Part model, mm, in its own coordinate system. Give positions to 0.01 mm unless a question says otherwise; leave off trailing zeros. Order: outer loops, then holes, each group sorted by start corner. A loop starts at its lowest first (then second) coordinate and runs counter-clockwise, first axis right, second up. Notation, with made-up numbers: (35.5, 5.5) -> (43.5, 5.5) arc R19 cw to (43.5, 38.5) -> close; hole circle Ø11 at (27.5, 7). An arc over 180 degrees is marked (long way). Write item = value, one per line. Start each with the question number.
(1) Probe line 1 along X through (y, z) = (0.35, 31.75); line 2 along X through (y, z) = (2.1, 31.75); line 3 along Z through (x, y) = (-5.08, 0.55). List the from-to ranges inside material, lowest first. Write a range as from..to.
(2) Saw through at C-C, the plane z = 31.75. State how many separate pieces and enclosed holes the cut face has, then the cut area to 3 significant figures.
(3) Saw through at A-A, the plane x = -68.5. List the corners of the cut face in (y, z) (3 decimals).
(4) Saw through at B-B, the plane z = 48. List the corners of the cut face in (x, y) (3 decimals), then the cut area to 3 significant figures.
(5) Saw through at D-D, the plane y = 7.25. List the corners of the cut face in (x, z) (3 decimals).
(6) Flat gauge pins, fed straight in: pin 1 (7.5 mm diameter, centred on x = -27.5, y = 10, fed in from -Z); pin 2 (2 mm diameter, centred on x = -23, y = 6.5, fed in from -Z); pin 3 (6 mm diameter, centred on x = -48, z = 8, fed in from +Y) (3 decimals). Where does each tip first touch, or does it go through?
Autodesk Inventor part; units mm, degrees
ref_plane "YZ Plane" through (0, 0, 0) normal (1, 0, 0) x (0, 1, 0)
ref_plane "XZ Plane" through (0, 0, 0) normal (0, 1, 0) x (-1, 0, 0)
ref_plane "XY Plane" through (0, 0, 0) normal (0, 0, 1) x (1, 0, 0)
sketch "Sketch1" plane through (0, 0, 0) normal (0, 1, 0) x (-1, 0, 0)
  line L0 (0, 0) -> (83.82, 0)
  line L1 (83.82, 0) -> (83.82, 63.5)
  line L2 (83.82, 63.5) -> (0, 63.5)
  line L3 (0, 63.5) -> (0, 0)
  line L4 (73.66, 53.975) -> (58.42, 53.975)
  line L5 (58.42, 53.975) -> (58.42, 9.525)
  line L6 (58.42, 9.525) -> (73.66, 9.525)
  line L7 (73.66, 9.525) -> (73.66, 53.975)
  line L8 (49.53, 53.975) -> (34.29, 53.975)
  line L9 (34.29, 53.975) -> (34.29, 9.525)
  line L10 (34.29, 9.525) -> (49.53, 9.525)
  line L11 (49.53, 9.525) -> (49.53, 53.975)
  line L12 (25.4, 53.975) -> (10.16, 53.975)
  line L13 (10.16, 53.975) -> (10.16, 9.525)
  line L14 (10.16, 9.525) -> (25.4, 9.525)
  line L15 (25.4, 9.525) -> (25.4, 53.975)
  dimension "d0" = 83.82
  dimension "d1" = 63.5
  dimension "d41" = 10.16
  dimension "d42" = 8.89
  dimension "d43" = 8.89
  dimension "d44" = 15.24
  dimension "d45" = 15.24
  dimension "d46" = 15.24
extrude "Extrusion1" add sketch "Sketch1" along normal blind 3.175
sketch "Sketch4" plane through (0, 3.175, 0) normal (0, 1, 0) x (1, 0, 0)
  line L0 (-83.82, -63.5) -> (0, -63.5)
  line L1 (0, 0) -> (-83.82, 0)
  line L2 (-66.675, 0) -> (-57.15, 0)
  line L3 (-57.15, 0) -> (-57.15, -3.9624)
  line L4 (-57.15, -3.9624) -> (-66.675, -3.9624)
  line L5 (-66.675, -3.9624) -> (-66.675, 0)
  line L6 (-31.75, 0) -> (-22.225, 0)
  line L7 (-22.225, 0) -> (-22.225, -3.9624)
  line L8 (-22.225, -3.9624) -> (-31.75, -3.9624)
  line L9 (-31.75, -3.9624) -> (-31.75, 0)
  line L10 (-66.675, -63.5) -> (-57.15, -63.5)
  line L11 (-57.15, -63.5) -> (-57.15, -59.5376)
  line L12 (-57.15, -59.5376) -> (-66.675, -59.5376)
  line L13 (-66.675, -59.5376) -> (-66.675, -63.5)
  line L14 (-31.75, -63.5) -> (-22.225, -63.5)
  line L15 (-22.225, -63.5) -> (-22.225, -59.5376)
  line L16 (-22.225, -59.5376) -> (-31.75, -59.5376)
  line L17 (-31.75, -59.5376) -> (-31.75, -63.5)
extrude "Extrusion4" add sketch "Sketch4" along normal blind 11.1252
sketch "Sketch5" plane through (-22.225, 3.175, 63.5) normal (1, 0, 0) x (0, 0, -1)
  line L0 (3.9624, 0) -> (0, 0)
  line L1 (3.9624, 0) -> (3.9624, 11.1252)
  line L2 (0, 11.1252) -> (3.9624, 11.1252)
  line L3 (0, 0) -> (0, 11.1252)
  line L4 (3.9624, 12.7) -> (2.1844, 12.7)
  line L5 (3.9624, -0.6232) -> (0.7874, -0.6232)
  line L6 (2.1844, 11.1252) -> (0.7874, 0)
  line L7 (0.7874, 0) -> (0, 0)
  line L8 (0, 0) -> (0, 11.1252)
  line L9 (0, 11.1252) -> (2.1844, 11.1252)
  line L10 (59.5376, 0) -> (63.5, 0)
  line L11 (59.5376, 0) -> (59.5376, 11.1252)
  line L12 (63.5, 11.1252) -> (59.5376, 11.1252)
  line L13 (63.5, 0) -> (63.5, 11.1252)
  line L14 (59.5376, 12.7) -> (61.3156, 12.7)
  line L15 (59.5376, -0.6232) -> (62.7126, -0.6232)
  line L16 (61.3156, 11.1252) -> (62.7126, 0)
  line L17 (62.7126, 0) -> (63.5, 0)
  line L18 (63.5, 0) -> (63.5, 11.1252)
  line L19 (63.5, 11.1252) -> (61.3156, 11.1252)
  point P0 (63.5, -3.175)
  dimension "d17" = 1.778
  dimension "d18" = 3.175
extrude "Extrusion5" cut sketch "Sketch5" against normal blind 44.45 contours L0 L3 L2 L6 | L16 L12 L13 L10
fillet "Fillet1" radius 3.175 4 edges at (-61.9125, 3.175, 62.7126) (-26.9875, 3.175, 62.7126) (-26.9875, 3.175, 0.7874) (-61.9125, 3.175, 0.7874)
sketch "Sketch6" plane through (0, 14.3002, 0) normal (0, 1, 0) x (1, 0, 0)
  line L0 (-22.225, -59.5376) -> (-31.75, -59.5376)
  line L1 (-31.75, -59.5376) -> (-22.225, -59.5376)
  line L2 (-22.225, -59.5376) -> (-22.225, -57.912)
  line L3 (-22.225, -57.912) -> (-31.75, -57.912)
  line L4 (-31.75, -57.912) -> (-31.75, -59.5376)
  line L5 (-57.15, -59.5376) -> (-66.675, -59.5376)
  line L6 (-66.675, -59.5376) -> (-66.675, -57.912)
  line L7 (-66.675, -57.912) -> (-57.15, -57.912)
  line L8 (-57.15, -57.912) -> (-57.15, -59.5376)
  line L9 (-31.75, -2.1844) -> (-22.225, -2.1844)
  line L10 (-22.225, -2.1844) -> (-22.225, -3.9624)
  line L11 (-22.225, -3.9624) -> (-31.75, -3.9624)
  line L12 (-31.75, -3.9624) -> (-31.75, -2.1844)
  line L13 (-31.75, -3.9624) -> (-22.225, -3.9624)
  line L14 (-22.225, -3.9624) -> (-22.225, -5.588)
  line L15 (-22.225, -5.588) -> (-31.75, -5.588)
  line L16 (-31.75, -5.588) -> (-31.75, -3.9624)
  line L17 (-57.15, -3.9624) -> (-66.675, -3.9624)
  line L18 (-66.675, -3.9624) -> (-66.675, -5.588)
  line L19 (-66.675, -5.588) -> (-57.15, -5.588)
  line L20 (-57.15, -5.588) -> (-57.15, -3.9624)
  line L21 (-66.675, -3.9624) -> (-57.15, -3.9624)
  point P0 (0, 0)
  dimension "d50" = 1.6256
  dimension "d51" = 1.6256
  dimension "d52" = 1.6256
  dimension "d53" = 1.6256
  dimension "d54" = 0
extrude "Extrusion6" add sketch "Sketch6" against normal blind 1.6002 contours L0 L4 L3 L2 | L5 L6 L7 L8 | L11 L14 L15 L16 | L20 L19 L18 L17
sketch "Sketch7" plane through (-22.225, 3.175, 63.5) normal (1, 0, 0) x (0, 0, -1)
  line L0 (5.588, 11.1252) -> (5.588, 9.525)
  line L1 (2.1844, 11.1252) -> (5.588, 11.1252)
  line L2 (4.5974, 11.1252) -> (5.588, 9.525)
  line L3 (4.5974, 11.1252) -> (5.588, 11.1252)
  line L4 (5.588, 9.525) -> (5.588, 11.1252)
  line L5 (61.3156, 11.1252) -> (62.4649, 1.9722)
  arc A0 (62.4649, 1.9722) -> (63.5, 0) centre (65.6152, 2.3678) ccw
  line L6 (59.5376, 0) -> (63.5, 0)
  line L7 (59.5376, 0) -> (59.5376, 9.525)
  line L8 (57.15, 9.525) -> (59.5376, 9.525)
  line L9 (57.15, 11.1252) -> (57.15, 9.525)
  line L10 (61.3156, 11.1252) -> (57.15, 11.1252)
  line L11 (58.9026, 11.1252) -> (57.15, 9.525)
  line L12 (58.9026, 11.1252) -> (57.15, 11.1252)
  line L13 (57.15, 9.525) -> (57.15, 11.1252)
  point P0 (63.5, -3.175)
extrude "Extrusion7" cut sketch "Sketch7" against normal blind 44.45 contours L0 L2 L1 | L11 L9 L10
sketch "Sketch8" plane through (0, 3.175, 0) normal (0, 1, 0) x (1, 0, 0)
  circle A0 centre (-79.0956, -31.75) radius 3.175
  circle A1 centre (-5.08, -31.75) radius 3.1695
  line L0 (0, -63.5) -> (0, 0)
  line L1 (-66.675, 0) -> (-83.82, 0)
  line L2 (0, 0) -> (-22.225, 0)
  dimension "d29" = 74.0156
  dimension "d47" = 5.08
  dimension "d48" = 31.75
  dimension "d49" = 31.75
extrude "Extrusion8" cut sketch "Sketch8" against normal blind 1.905
sketch "Sketch9" plane through (0, 3.175, 0) normal (0, 1, 0) x (1, 0, 0)
  circle A0 centre (-5.08, -31.75) radius 3.1695
  circle A1 centre (-79.0956, -31.75) radius 3.175
  circle A2 centre (-79.0956, -31.75) radius 1.5875
  circle A3 centre (-5.08, -31.75) radius 1.5875
extrude "Extrusion9" cut sketch "Sketch9" against normal blind 3.175 contours A2 | A3
sketch "Sketch12" plane through (0, 12.7, 0) normal (0, -1, 0) x (1, 0, 0)
  line L0 (-22.225, 3.9624) -> (-22.225, 5.588)
  line L1 (-22.225, 5.588) -> (-31.75, 5.588)
  line L2 (-22.225, 3.9624) -> (-31.75, 3.9624)
  line L3 (-31.75, 3.9624) -> (-31.75, 5.588)
  line L4 (-31.75, 5.588) -> (-22.225, 5.588)
  line L5 (-22.225, 5.588) -> (-22.225, 3.9624)
  line L6 (-57.15, 3.9624) -> (-66.675, 3.9624)
  line L7 (-57.15, 5.588) -> (-66.675, 5.588)
  line L8 (-57.15, 3.9624) -> (-66.675, 3.9624)
  line L9 (-66.675, 3.9624) -> (-66.675, 5.588)
  line L10 (-66.675, 5.588) -> (-57.15, 5.588)
  line L11 (-57.15, 5.588) -> (-57.15, 3.9624)
  line L12 (-66.675, 57.912) -> (-57.15, 57.912)
  line L13 (-57.15, 59.5376) -> (-66.675, 59.5376)
  line L14 (-66.675, 59.5376) -> (-66.675, 57.912)
  line L15 (-66.675, 57.912) -> (-57.15, 57.912)
  line L16 (-57.15, 57.912) -> (-57.15, 59.5376)
  line L17 (-31.75, 57.912) -> (-22.225, 57.912)
  line L18 (-31.75, 59.5376) -> (-22.225, 59.5376)
  line L19 (-22.225, 57.912) -> (-31.75, 57.912)
  line L20 (-31.75, 57.912) -> (-31.75, 59.5376)
  line L21 (-31.75, 59.5376) -> (-22.225, 59.5376)
  line L22 (-22.225, 59.5376) -> (-22.225, 57.912)
  point P0 (0, 0)
equation "\"d43\" = d42"
equation "\"d45\" = d44"
equation "\"d46\" = d44"
equation "\"d51\" = d50"
equation "\"d52\" = d50"
equation "\"d53\" = d50"
properties part number "_3DPrint"
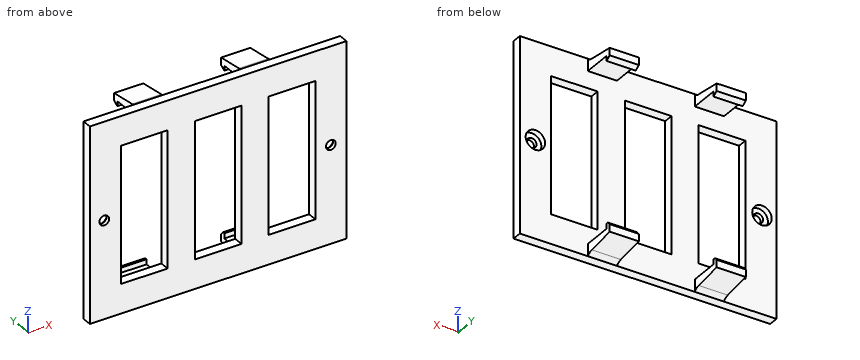
Results list:
q1.line_1 = -83.82..-80.68, -77.51..-73.66, -58.42..-49.53, -34.29..-25.4, -10.16..-6.67, -3.49..0
q1.line_2 = -83.82..-82.27, -75.92..-73.66, -58.42..-49.53, -34.29..-25.4, -10.16..-8.25, -1.91..0
q1.line_3 = 0..30.16, 33.34..63.5
q2.separate_pieces = 6
q2.enclosed_holes = 0
q2.area = 88.7 mm^2
q3.outline = (0, 0) -> (3.175, 0) -> (3.175, 9.525) -> (0, 9.525) -> close; (0, 53.975) -> (3.175, 53.975) -> (3.175, 63.5) -> (0, 63.5) -> close
q4.outline = (-83.82, 0) -> (-73.66, 0) -> (-73.66, 3.175) -> (-83.82, 3.175) -> close; (-58.42, 0) -> (-49.53, 0) -> (-49.53, 3.175) -> (-58.42, 3.175) -> close; (-34.29, 0) -> (-25.4, 0) -> (-25.4, 3.175) -> (-34.29, 3.175) -> close; (-10.16, 0) -> (0, 0) -> (0, 3.175) -> (-10.16, 3.175) -> close
q4.area = 121 mm^2
q5.outline = (-66.675, 1.299) -> (-57.15, 1.299) -> (-57.15, 3.962) -> (-66.675, 3.962) -> close; (-66.675, 59.538) -> (-57.15, 59.538) -> (-57.15, 62.201) -> (-66.675, 62.201) -> close; (-31.75, 1.299) -> (-22.225, 1.299) -> (-22.225, 3.962) -> (-31.75, 3.962) -> close; (-31.75, 59.538) -> (-22.225, 59.538) -> (-22.225, 62.201) -> (-31.75, 62.201) -> close
q6.pin_1 = 1.17
q6.pin_2 = 1.08
q6.pin_3 = 3.175
